Source: CAD feature listing. Evaluate the final solid. Frame: model axes, mm. Coordinates: 2 decimals unless noted, no trailing zeros. Write each loop counter-clockwise with the first axis right and the second up, starting at its lowest first coordinate (ties: lowest second). Pieces come first, ordered by that corner, then holes. Notation, with made-up numbers: M 33.25,14.25 L 91.25,14.25 A20 cw 91.25,36.25 Z; hole C 30,-27.5 d5. An arc over 180 degrees is marked long. Write item = value, one per line. Start each with the question number.
1. Section query C-C (x = -21.9). Output: boundary loops of the cut face in (y, z), then the cut area to 3 significant figures.
2. Pin query (flat end, axial travel): pin 1 Ø1.6 at (x, y) = (0, 14.9) entering from +Z. Return the tip coordinate at first contact, or that it passes through.
3. Section query B-B (y = -14.9). Output: boundary loops of the cut face in (x, z), then the cut area to 3 significant figures.
4. Section query A-A (z = 2.5). Output: boundary loops of the cut face in (x, y), then the cut area to 3 significant figures.
5. Line query: line 1 along Y through (x, z) = (-21.9, 2.05); line 2 along X through (y, z) = (15, 0.25). Output: solid intervals per line, ascending.
```python
from build123d import *

# Parameters (mm, degrees)
ESBO_O1_W                = 49
ESBO_O1_H                = 35
RESSALTO_EXTRUS_O1_DEPTH = 3
ESBO_O2_R                = 1.35
CORTE_EXTRUS_O1_DEPTH    = 31.257230541
ESBO_O3_W                = 49
ESBO_O3_H                = 3
RESSALTO_EXTRUS_O3_DEPTH = 8
ESBO_O4_R                = 1.35
CORTE_EXTRUS_O2_DEPTH    = 44.465503563
FILETE1_R                = 2
FILETE2_R                = 2
CORTE_EXTRUS_O3_DEPTH    = 10
FILETE3_R                = 2
ESBO_O6_R                = 1.35
CORTE_EXTRUS_O4_DEPTH    = 31.257230541


with BuildPart() as part:
    # Esboço1 → Ressalto-extrusão1 (new body)
    with BuildSketch(Plane.XY):
        Rectangle(ESBO_O1_W, ESBO_O1_H)
    extrude(amount=RESSALTO_EXTRUS_O1_DEPTH)

    # Esboço2 → Corte-extrusão1 (cut, through all)
    with BuildSketch(Plane(origin=(0, 0, 0), x_dir=(-1, 0, 0), z_dir=(0, 0, -1))):
        with Locations((-21.9, -14.9)):
            Circle(ESBO_O2_R)
        with Locations((0, -14.9)):
            Circle(ESBO_O2_R)
        with Locations((21.9, -14.9)):
            Circle(ESBO_O2_R)
    extrude(amount=-CORTE_EXTRUS_O1_DEPTH, mode=Mode.SUBTRACT)

    # Esboço3 → Ressalto-extrusão3 (add)
    with BuildSketch(Plane(origin=(0, 0, 0), x_dir=(-1, 0, 0), z_dir=(0, 0, -1))):
        with Locations((0, 16)):
            Rectangle(ESBO_O3_W, ESBO_O3_H)
    extrude(amount=RESSALTO_EXTRUS_O3_DEPTH)

    # Esboço4 → Corte-extrusão2 (cut, through all)
    with BuildSketch(Plane(origin=(0, 17.5, 0), x_dir=(1, 0, 0), z_dir=(0, 1, 0))):
        with Locations(Location((-21.9, 5.4, 0), (0, 0, 270))):
            Circle(ESBO_O4_R)
        with Locations(Location((0, 5.4, 0), (0, 0, 270))):
            Circle(ESBO_O4_R)
        with Locations(Location((21.9, 5.4, 0), (0, 0, 270))):
            Circle(ESBO_O4_R)
    extrude(amount=-CORTE_EXTRUS_O2_DEPTH, mode=Mode.SUBTRACT)

    # Filete1
    filete1_edges = [part.edges().sort_by_distance(p)[0] for p in [
        (24.5, -17.5, 1.5),
        (-24.5, -17.5, 1.5),
    ]]
    fillet(filete1_edges, radius=FILETE1_R)

    # Filete2
    filete2_edges = [part.edges().sort_by_distance(p)[0] for p in [
        (24.5, 16, -8),
        (-24.5, 16, -8),
    ]]
    fillet(filete2_edges, radius=FILETE2_R)

    # Esboço5 → Corte-extrusão3 (cut)
    with BuildSketch(Plane(origin=(0, 14.5, 0), x_dir=(-1, 0, 0), z_dir=(0, -1, 0))):
        Polygon((24.5, 0), (24.5, 8), (22.5, 8), (-24.5, 8), (-24.5, 0), align=None)
    extrude(amount=-CORTE_EXTRUS_O3_DEPTH, mode=Mode.SUBTRACT)

    # Filete3
    filete3_edges = [part.edges().sort_by_distance(p)[0] for p in [
        (-24.5, 17.5, 1.5),
        (24.5, 17.5, 1.5),
    ]]
    fillet(filete3_edges, radius=FILETE3_R)

    # Esboço6 → Corte-extrusão4 (cut, through all)
    with BuildSketch(Plane.XY.offset(3)):
        with Locations((21.9, 14.9)):
            Circle(ESBO_O6_R)
        with Locations((0, 14.9)):
            Circle(ESBO_O6_R)
        with Locations((-21.9, 14.9)):
            Circle(ESBO_O6_R)
    extrude(amount=-CORTE_EXTRUS_O4_DEPTH, mode=Mode.SUBTRACT)


solid = part.part
```
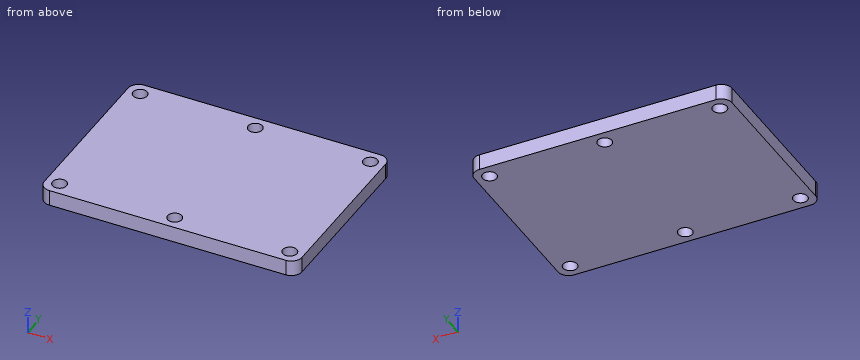
Results are:
q1.outline = M -17.5,0 L -16.25,0 L -16.25,3 L -17.5,3 Z; M -13.55,0 L 13.55,0 L 13.55,3 L -13.55,3 Z; M 16.25,0 L 17.5,0 L 17.5,3 L 16.25,3 Z
q1.area = 88.8 mm^2
q2.pin_1 = through
q3.outline = M -24.5,0 L -23.25,0 L -23.25,3 L -24.5,3 Z; M -20.55,0 L -1.35,0 L -1.35,3 L -20.55,3 Z; M 1.35,0 L 20.55,0 L 20.55,3 L 1.35,3 Z; M 23.25,0 L 24.5,0 L 24.5,3 L 23.25,3 Z
q3.area = 123 mm^2
q4.outline = M -24.5,-15.5 A2 ccw -22.5,-17.5 L 22.5,-17.5 A2 ccw 24.5,-15.5 L 24.5,15.5 A2 ccw 22.5,17.5 L -22.5,17.5 A2 ccw -24.5,15.5 Z; hole C -21.9,-14.9 d2.7; hole C -21.9,14.9 d2.7; hole C 0,-14.9 d2.7; hole C 0,14.9 d2.7; hole C 21.9,-14.9 d2.7; hole C 21.9,14.9 d2.7
q4.area = 1,680 mm^2
q5.line_1 = -17.5 to -16.25, -13.55 to 13.55, 16.25 to 17.5
q5.line_2 = -24.5 to -23.25, -20.55 to -1.35, 1.35 to 20.55, 23.25 to 24.5
